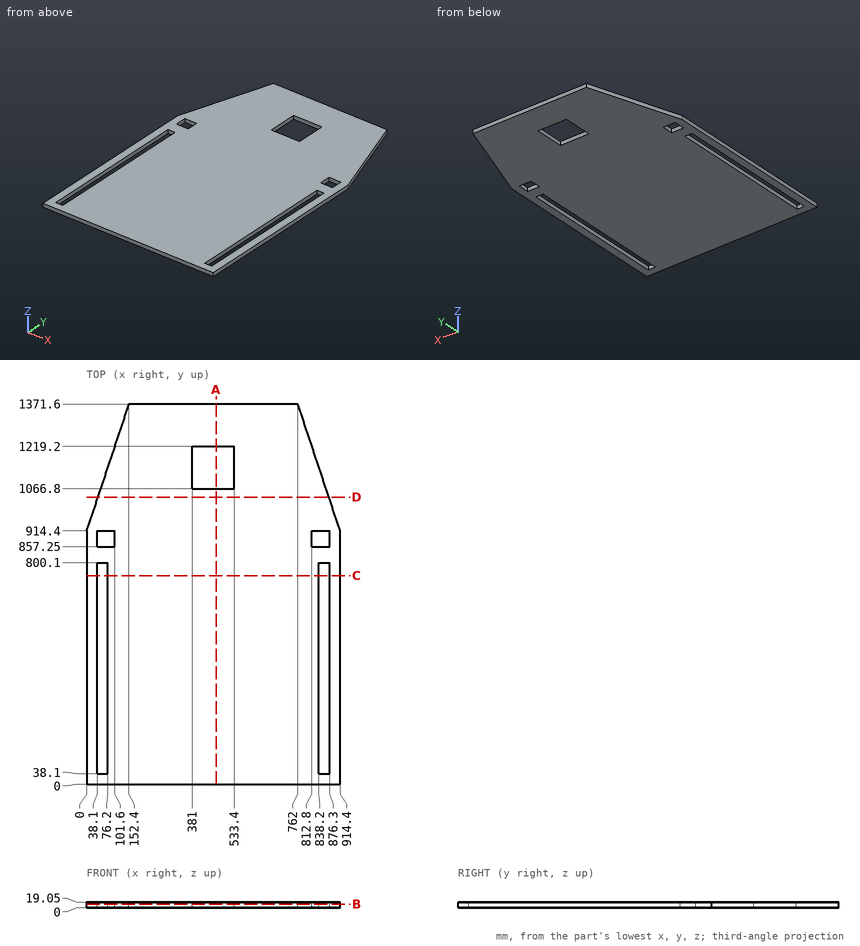
Verification items for this drawing (mm, ordinates from the low corner). Coordinates: 2 decimals unless noted, no trailing zeros. Write each loop counter-clockwise with the first axis right and the second up, starting at its lowest first coordinate (ties: lowest second). Pieces come first, ordered by that corner, then holes. Notation, with made-up numbers: M -33,16.5 L -19,16.5 A19 ccw -19,44.5 Z; hole C -25,6.25 d4. An arc over 180 degrees is marked long. Answer as a JSON object with one key per item and string values. Group by question number.
(1) Cross-section at A-A, the plane x = 467.5. Record the cut outline in (y, z), and give its area (3 significant figures).
(2) Gauge pin test, flat ends, axial feed: pin 1 (3 mm diameter, centred on y = 997.5, z = 14.5, fed in from -X); pin 2 (3 mm diameter, centred on y = 1167.5, z = 16.5, fed in from +X). Record the tip position at first contact, or that the pin passes through.
(3) Cross-section at B-B, the plane z = 12.75. Record the cut outline in (x, y), and give its area (3 significant figures).
(4) Cross-section at D-D, the plane y = 1035.5. Record the cut outline in (x, z), and give its area (3 significant figures).
(5) Cross-section at C-C, the plane y = 753. Record the cut outline in (x, z).
(6) Material ranges on line 1 (X direction, y = 897, z = 2.25); line 2 (X direction, y = 156, z = 4); line 3 (Y direction, x = 415.5, z = 10.75), recorded low to high.
Reply:
{
 "1": {"outline": "M 0,0 L 1066.8,0 L 1066.8,19.05 L 0,19.05 Z; M 1219.2,0 L 1371.6,0 L 1371.6,19.05 L 1219.2,19.05 Z", "area": "23,200 mm²"},
 "2": {"pin 1": "x = 27.2", "pin 2": "x = 830.53"},
 "3": {"outline": "M 0,0 L 914.4,0 L 914.4,914.4 L 762,1371.6 L 152.4,1371.6 L 0,914.4 Z; hole M 38.1,38.1 L 76.2,38.1 L 76.2,800.1 L 38.1,800.1 Z; hole M 38.1,857.25 L 101.6,857.25 L 101.6,914.4 L 38.1,914.4 Z; hole M 381,1066.8 L 533.4,1066.8 L 533.4,1219.2 L 381,1219.2 Z; hole M 812.8,857.25 L 876.3,857.25 L 876.3,914.4 L 812.8,914.4 Z; hole M 838.2,38.1 L 876.3,38.1 L 876.3,800.1 L 838.2,800.1 Z", "area": "1,100,000 mm²"},
 "4": {"outline": "M 40.37,0 L 874.03,0 L 874.03,19.05 L 40.37,19.05 Z", "area": "15,900 mm²"},
 "5": {"outline": "M 0,0 L 38.1,0 L 38.1,19.05 L 0,19.05 Z; M 76.2,0 L 838.2,0 L 838.2,19.05 L 76.2,19.05 Z; M 876.3,0 L 914.4,0 L 914.4,19.05 L 876.3,19.05 Z"},
 "6": {"line 1": "0 to 38.1, 101.6 to 812.8, 876.3 to 914.4", "line 2": "0 to 38.1, 76.2 to 838.2, 876.3 to 914.4", "line 3": "0 to 1066.8, 1219.2 to 1371.6"}
}
